Autodesk Inventor part; units mm, degrees
ref_plane "YZ Plane" through (0, 0, 0) normal (1, 0, 0) x (0, 1, 0)
ref_plane "XZ Plane" through (0, 0, 0) normal (0, 1, 0) x (-1, 0, 0)
ref_plane "XY Plane" through (0, 0, 0) normal (0, 0, 1) x (1, 0, 0)
sketch "スケッチ1" plane through (0, 0, 0) normal (0, 0, 1) x (1, 0, 0)
  line L0 (-24.13, -13.97) -> (24.13, -13.97)
  line L1 (24.13, -13.97) -> (24.13, 13.97)
  line L2 (24.13, 13.97) -> (-24.13, 13.97)
  line L3 (-24.13, 13.97) -> (-24.13, -13.97)
  point P0 (0, 0)
  point P1 (0, -13.97)
  point P2 (24.13, 0)
  dimension "d0" = 48.26
  dimension "d1" = 27.94
extrude "押し出し1" add sketch "スケッチ1" along normal blind 1.3
sketch "スケッチ2" plane through (0, 0, 1.3) normal (0, 0, 1) x (1, 0, 0)
  line L0 (-24.13, 13.97) -> (-24.13, -13.97)
  line L1 (24.13, 13.97) -> (-24.13, 13.97)
  line L2 (-24.13, -13.97) -> (24.13, -13.97)
  line L3 (24.13, -13.97) -> (24.13, 13.97)
  circle A0 centre (-20.32, 10.16) radius 1.5
  circle A1 centre (-20.32, -10.16) radius 1.5
  circle A2 centre (20.32, -10.16) radius 1.5
  circle A3 centre (20.32, 10.16) radius 1.5
  point P0 (0, 0)
  dimension "d4" = 3.81
  dimension "d5" = 3.81
  dimension "d6" = 3.81
  dimension "d7" = 3.81
  dimension "d8" = 3
extrude "押し出し2" cut sketch "スケッチ2" against normal blind 1.3 contours A0 | A1 | A2 | A3
sketch "スケッチ3" plane through (0, 0, 1.3) normal (0, 0, 1) x (1, 0, 0)
  circle A0 centre (-20.32, -10.16) radius 1.5
  line L0 (-1.27, -8.89) -> (-3.81, -8.89)
  line L1 (-3.81, -8.89) -> (-3.81, 3.81)
  line L2 (-3.81, 3.81) -> (-1.27, 3.81)
  line L3 (-1.27, 3.81) -> (-1.27, -8.89)
  point P0 (0, 0)
  point P1 (-2.54, -7.62)
  point P2 (-2.54, -8.89)
  dimension "d11" = 17.78
  dimension "d12" = 2.54
  dimension "d13" = 2.54
  dimension "d14" = 12.7
  dimension "d15" = 1.27
extrude "押し出し3" add sketch "スケッチ3" along normal blind 8.5 contours L0 L1 L2 L3
sketch "スケッチ4" plane through (0, 0, 9.8) normal (0, 0, 1) x (1, 0, 0)
  line L0 (-3.81, 3.81) -> (-1.27, 3.81)
  line L1 (-1.27, 3.81) -> (-1.27, -8.89)
  line L2 (-1.27, -8.89) -> (-3.81, -8.89)
  line L3 (-3.81, -8.89) -> (-3.81, 3.81)
  point P0 (0, 0)
extrude "押し出し4" add sketch "スケッチ4" along normal blind 2
sketch "スケッチ5" plane through (0, 0, 11.8) normal (0, 0, 1) x (1, 0, 0)
  line L0 (-5.35, 8.46) -> (29.65, 8.46)
  line L1 (29.65, 8.46) -> (29.65, -13.54)
  line L2 (29.65, -13.54) -> (-5.35, -13.54)
  line L3 (-5.35, -13.54) -> (-5.35, 8.46)
  line L4 (-3.81, 3.81) -> (-3.81, -8.89)
  point P0 (0, 0)
  point P1 (-5.35, -2.54)
  point P2 (-3.81, -2.54)
  dimension "d20" = 35
  dimension "d21" = 22
  dimension "d22" = 1.54
extrude "押し出し5" add sketch "スケッチ5" along normal blind 1.2
sketch "スケッチ6" plane through (0, 0, 13) normal (0, 0, 1) x (1, 0, 0)
  line L0 (29.15, 6.96) -> (-0.85, 6.96)
  line L1 (-0.85, 6.96) -> (-0.85, -12.54)
  line L2 (-0.85, -12.54) -> (29.15, -12.54)
  line L3 (29.15, -12.54) -> (29.15, 6.96)
  line L4 (29.65, -13.54) -> (29.65, 8.46)
  point P0 (0, 0)
  dimension "d25" = 30
  dimension "d26" = 19.5
  dimension "d27" = 0.5
  dimension "d28" = 1
extrude "押し出し6" add sketch "スケッチ6" along normal blind 2
properties part number "LCD-RTC"
Could you check a few things on this model? Use its own coordinates, in mm. A direction names the side the tool comes from. Give positions to 0.01 mm unless a question says otherwise; leave off trailing zeros. Write each loop counter-clockwise with the first axis right and the second up, starting at its lowest first coordinate (ties: lowest second). Pieces come first, ordered by that corner, then holes. Notation, with made-up numbers: (77.5, 44.25) -> (129.5, 44.25) arc R27 cw to (129.5, 73.25) -> close; hole circle Ø3 at (42, 36.5). An arc over 180 degrees is marked (long way). Write each question's results on one line, items separated by ' | '. Start each with the question number.
Q1. Suppose I cut it at C-C, the plane y = -10.16. List the corners of the cut face in (x, z) for me, and give its area (3 significant figures).
Q2. I'm going to push flat-ended pins straight in: pin 1 Ø0.6 at (x, z) = (3.5, 12) entering from +Y; pin 2 Ø5 at (x, y) = (-18, 9.5) entering from -Z; pin 3 Ø0.6 at (x, z) = (21.5, 13.5) entering from -Y; pin 4 Ø1.3 at (x, z) = (-2, 5) entering from +Y. Where does each tip first touch, or does it pass through?
Q3. Which directions (+Z, -Z, +X, -X, +Y, -Y) give clear straight access to the entire face, cutting with the end or side of a thin tool? Please do faces 1 (the face through (-0.85, -3, 14)), 2 (the face through (-3, 3.81, 6)), 3 (the face through (14, 6.96, 14)), 4 (the face through (-3.81, -3, 6)).
Q4. We'd pull the mould along Y, two halves only. Please class faces 5 (the face through (-3, -8.89, 6)), 6 (the face through (-18.934, 9.585, 0.659)), 7 (the face through (29.15, -3, 14)), 8 (the face through (12, 8.46, 12)): +Y half, -Y half, draft (parallel to the pull), parting line (faces both ways), or undercut.
Q5. I need wall thicknesses on probe 1 along Y at (x, z) = (20.32, 0.8); probe 2 along Z at (x, y) = (14, 5.5); probe 3 along Z at (x, y) = (-7, 9.5). Which ranges of each line are inside material? Lowest first, please.
Q6. Suppose I cut it at A-A, the plane y = 10.16. List the corners of the cut face in (x, z) for me, and give its area (3 significant figures).
Q7. Suppose I cut it at B-B, the plane x = 20.32. List the corners of the cut face in (y, z) for me, and give its area (3 significant figures).
Q8. Suppose I cut it at D-D, the plane x = -20.32. List the corners of the cut face in (y, z) for me.
Outcome:
1) outline: (-24.13, 0) -> (-21.82, 0) -> (-21.82, 1.3) -> (-24.13, 1.3) -> close; (-18.82, 0) -> (18.82, 0) -> (18.82, 1.3) -> (-18.82, 1.3) -> close; (-5.35, 11.8) -> (29.65, 11.8) -> (29.65, 13) -> (29.15, 13) -> (29.15, 15) -> (-0.85, 15) -> (-0.85, 13) -> (-5.35, 13) -> close; (21.82, 0) -> (24.13, 0) -> (24.13, 1.3) -> (21.82, 1.3) -> close | area: 157 mm2
2) pin 1: y = 8.46 | pin 2: z = 0 | pin 3: y = -12.54 | pin 4: y = 3.81
3) face 1: +Z, -X, +Y, -Y | face 2: +X, -X, +Y | face 3: +Z, +X, -X, +Y | face 4: -X, +Y, -Y
4) face 5: -Y half | face 6: undercut | face 7: draft | face 8: +Y half
5) probe 1: -13.97 to -11.66, -8.66 to 8.66, 11.66 to 13.97 | probe 2: 0 to 1.3, 11.8 to 15 | probe 3: 0 to 1.3
6) outline: (-24.13, 0) -> (-21.82, 0) -> (-21.82, 1.3) -> (-24.13, 1.3) -> close; (-18.82, 0) -> (18.82, 0) -> (18.82, 1.3) -> (-18.82, 1.3) -> close; (21.82, 0) -> (24.13, 0) -> (24.13, 1.3) -> (21.82, 1.3) -> close | area: 54.9 mm2
7) outline: (-13.97, 0) -> (-11.66, 0) -> (-11.66, 1.3) -> (-13.97, 1.3) -> close; (-13.54, 11.8) -> (8.46, 11.8) -> (8.46, 13) -> (6.96, 13) -> (6.96, 15) -> (-12.54, 15) -> (-12.54, 13) -> (-13.54, 13) -> close; (-8.66, 0) -> (8.66, 0) -> (8.66, 1.3) -> (-8.66, 1.3) -> close; (11.66, 0) -> (13.97, 0) -> (13.97, 1.3) -> (11.66, 1.3) -> close | area: 93.9 mm2
8) outline: (-13.97, 0) -> (-11.66, 0) -> (-11.66, 1.3) -> (-13.97, 1.3) -> close; (-8.66, 0) -> (8.66, 0) -> (8.66, 1.3) -> (-8.66, 1.3) -> close; (11.66, 0) -> (13.97, 0) -> (13.97, 1.3) -> (11.66, 1.3) -> close
